CAD build for the part. Positions are in the model's coordinates, mm. A direction names the side the tool comes from. Coordinates: 2 decimals unless noted, no trailing zeros. Loops run counter-clockwise (first coordinate to the right, second up) from the corner with the lowest first, then second, coordinate; pieces in that order, holes last. Notation, with made-up numbers: (73.25, 49.5) - (92.25, 49.5) arc R25 ccw to (92.25, 83.5) - close; hole circle Ø3 at (-11, -3.75). An arc over 180 degrees is marked (long way). Put each result on its own line as item: value.
```python
from build123d import *

# Parameters (mm, degrees)
SKETCH1_R               = 3.175
BOSS_EXTRUDE1_DEPTH     = 50.8
CUT_EXTRUDE1_DEPTH      = 64.844432524
CUT_EXTRUDE1_DEPTH_BACK = 64.844432524
SKETCH2_W               = 10.868428171
SKETCH2_H               = 12.7
SKETCH2_H_2             = 12.700000009


with BuildPart() as part:
    # Sketch1 → Boss-Extrude1 (new body)
    with BuildSketch(Plane.XY):
        with BuildLine():
            Line((1.143472567, 262.725830005), (-38.1, 262.725830005))
            Line((-38.1, 262.725830005), (-38.1, 268.577174682))
            Line((-38.1, 268.577174682), (-2.377184588, 268.577174682))
            ThreePointArc((-2.377184588, 268.577174682), (9.92041245, 271.991602208), (1.143472567, 262.725830005))
        make_face()
        with Locations((4.245621792, 268.577174682)):
            Circle(SKETCH1_R, mode=Mode.SUBTRACT)
    extrude(amount=-BOSS_EXTRUDE1_DEPTH)

    # Sketch2 → Cut-Extrude1 (cut, two sides: drawn at the far end of the back side and taken through both)
    with BuildSketch(Plane(origin=(0, 268.577174682, 0), x_dir=(1, 0, 0), z_dir=(0, 1, 0)).offset(-CUT_EXTRUDE1_DEPTH_BACK)):
        with Locations((5.434214086, 19.05)):
            Rectangle(SKETCH2_W, SKETCH2_H)
        with Locations((5.434214086, 44.449999996)):
            Rectangle(SKETCH2_W, SKETCH2_H_2)
    extrude(amount=CUT_EXTRUDE1_DEPTH + CUT_EXTRUDE1_DEPTH_BACK, mode=Mode.SUBTRACT)


solid = part.part
```
Q1. Mould opens along X. For faces 1 (the cylindrical face through (3.557, 265.478, -6.261)), 2 (the flat face through (-20, 268.577, -25)), 3 (the flat face through (0, 268, -44)) say: +X half, -X half, draft (parallel to the pull), parting line (faces both ways), or undercut.
Determined:
face 1: undercut
face 2: draft
face 3: +X half
Q2. Slice it at B-B, the plane z = -24.5. Give the cut face in (x, y), then the cut area to 3 significant figures.
Determined:
outline: (-38.1, 262.73) - (0, 262.73) - (0, 273.66) arc R6.62 ccw to (-2.38, 268.58) - (-38.1, 268.58) - close
area: 231 mm2
Q3. Slice it at D-D, the plane y = 274.5. Give the cut face in (x, z).
Determined:
outline: (1.28, -38.1) - (7.21, -38.1) - (7.21, -25.4) - (1.28, -25.4) - close; (1.28, -12.7) - (7.21, -12.7) - (7.21, 0) - (1.28, 0) - close
Q4. Slice it at A-A, the plane y = 271. Give the cut face in (x, z), then the cut area to 3 significant figures.
Determined:
outline: (-1.92, -50.8) - (0, -50.8) - (0, -38.1) - (2.19, -38.1) - (2.19, -25.4) - (0, -25.4) - (0, -12.7) - (2.19, -12.7) - (2.19, 0) - (-1.92, 0) - close; (6.3, -38.1) - (10.41, -38.1) - (10.41, -25.4) - (6.3, -25.4) - close; (6.3, -12.7) - (10.41, -12.7) - (10.41, 0) - (6.3, 0) - close
area: 258 mm2
Q5. Slice it at C-C, the plane x = 5. Give the cut face in (y, z).
Determined:
outline: (262, -38.1) - (265.49, -38.1) - (265.49, -25.4) - (262, -25.4) - close; (262, -12.7) - (265.49, -12.7) - (265.49, 0) - (262, 0) - close; (271.66, -38.1) - (275.16, -38.1) - (275.16, -25.4) - (271.66, -25.4) - close; (271.66, -12.7) - (275.16, -12.7) - (275.16, 0) - (271.66, 0) - close
Q6. Wall check: L1, parallel to Y at x = -17.5, z = -30; L2, parallel to X at y = 264.25, z = -48; L3, parallel to X at y = 266, z = -9. Give the ranges that are in metal, low to high. Write a range as from..to.
Determined:
L1: 262.73..268.58
L2: -38.1..0
L3: -38.1..2.39, 6.1..10.35
Q7. Pin check, flat tips, straight feed: pin 1 Ø18 at (x, z) = (-23.5, -23.5) entering from +Y; pin 2 Ø3.5 at (y, z) = (267, -19.5) entering from +X; pin 3 Ø5.5 at (x, y) = (5.5, 265.5) entering from -Z. Stop position of each tip, or through.
Determined:
pin 1: y = 268.58
pin 2: x = 0
pin 3: z = -38.1
Q8. Tool access for faces 4 (the flat face through (-18, 262.726, -25)), 5 (the flat face through (8, 268, -38.1)), 6 (the flat face through (8, 268, -25.4)): list every direction of +Z, -Z, +X, -X, +Y, -Y with a clear straight run to the whole face (end or side of a thin tool).
Determined:
face 4: +Z, -Z, -X, -Y
face 5: -Z, +X, +Y, -Y
face 6: +X, +Y, -Y
